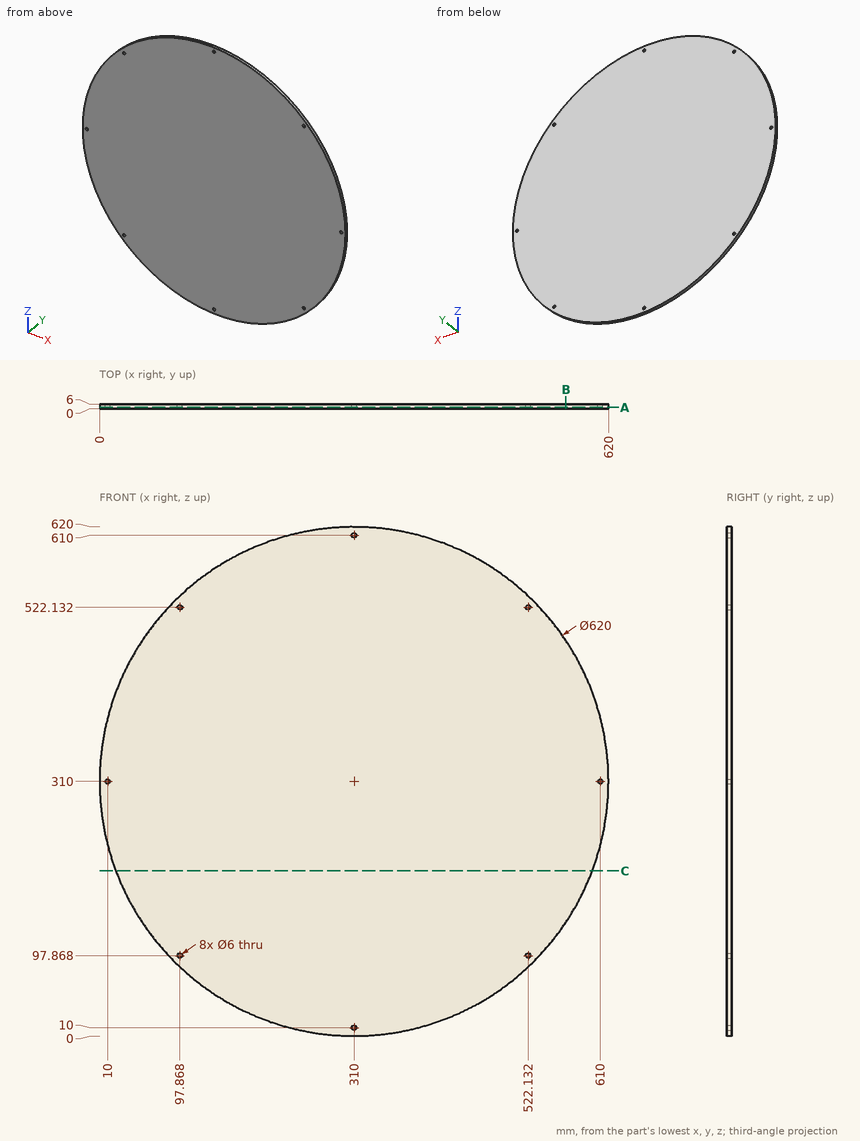
Answer from the drawing. Dimensions are ordinates in mm from the lowest x, y and z of the part. Round coordinates to 2 decimals unless told otherwise and drop trailing zeros. Write each loop counter-clockwise with the first axis right and the second up, starting at its lowest first coordinate (ties: lowest second). Pieces come first, ordered by that corner, then holes. Notation, with made-up numbers: (-9, 62.5) -> (20, 62.5) arc R26 cw to (20, 90.5) -> close; hole circle Ø6 at (56, -2.5). An arc over 180 degrees is marked (long way). Answer in a Markdown table with one row per item. Add a question column.
1) Consider line 1 (Z direction, x = 310, y = 4.75); line 2 (Z direction, x = 245, y = 2.5); line 3 (X direction, y = 2.4, z = 423). Determine where each line is inside the solid, lowest interval first.
2) Find section A-A, the plane y = 1.8. State how many separate pieces and enclosed holes the cut face has, and give its area (3 significant figures).
3) Given P1, Ø1.5, axis at y = 0.5, z = 504.5, coming from the +X side; P2, Ø1, axis at x = 398.5, y = 4, coming from the +Z side; P3, Ø1, axis at y = 3.5, z = 266.5, coming from the -X side, each flat-ended and moving along its own axis, determine where each tip first touches the part or whether it passes through.
4) Find section B-B, the plane x = 568. Determine the outline of the cut face in (y, z), and give its area (3 significant figures).
5) Find section C-C, the plane z = 201. Determine the outline of the cut face in (x, y).
Findings below:
| question | item | result |
|---|---|---|
| 1 | line 1 | 0 to 7, 13 to 607, 613 to 620 |
| 1 | line 2 | 6.89 to 613.11 |
| 1 | line 3 | 21.33 to 598.67 |
| 2 | separate pieces | 1 |
| 2 | enclosed holes | 8 |
| 2 | area | 302,000 mm² |
| 3 | P1 | x = 551.99 |
| 3 | P2 | z = 607.25 |
| 3 | P3 | x = 3 |
| 4 | outline | (0, 138.14) -> (6, 138.14) -> (6, 481.86) -> (0, 481.86) -> close |
| 4 | area | 2,060 mm² |
| 5 | outline | (19.79, 0) -> (600.21, 0) -> (600.21, 6) -> (19.79, 6) -> close |
